```python
from build123d import *

# Parameters (mm, degrees)
SKETCH1_W           = 44
SKETCH1_H           = 29
BOSS_EXTRUDE1_DEPTH = 10.2
SKETCH2_W           = 8
SKETCH2_H           = 4
BOSS_EXTRUDE2_DEPTH = 4.3
FILLET1_R           = 3


with BuildPart() as part:
    # Sketch1 → Boss-Extrude1 (new body)
    with BuildSketch(Plane(origin=(0, 0, 0), x_dir=(1, 0, 0), z_dir=(0, 1, 0))):
        with Locations((22, 14.5)):
            Rectangle(SKETCH1_W, SKETCH1_H)
    extrude(amount=BOSS_EXTRUDE1_DEPTH)

    # Sketch2 → Boss-Extrude2 (add)
    with BuildSketch(Plane(origin=(0, 10.2, 0), x_dir=(1, 0, 0), z_dir=(0, 1, 0))):
        with Locations((28.5, 2)):
            Rectangle(SKETCH2_W, SKETCH2_H)
        with Locations((15.5, 2)):
            Rectangle(SKETCH2_W, SKETCH2_H)
    extrude(amount=BOSS_EXTRUDE2_DEPTH)

    # Fillet1
    fillet1_edges = [part.edges().sort_by_distance(p)[0] for p in [
        (0, 5.1, -29),
        (44, 5.1, -29),
        (44, 5.1, 0),
        (0, 5.1, 0),
    ]]
    fillet(fillet1_edges, radius=FILLET1_R)


solid = part.part
```
The model under review builds one solid part; all positions refer to its coordinate system, in mm. A direction names the side the tool comes from. Give positions to 0.01 mm unless a question says otherwise; leave off trailing zeros. Write each loop counter-clockwise with the first axis right and the second up, starting at its lowest first coordinate (ties: lowest second). Pieces come first, ordered by that corner, then holes. Notation, with made-up numbers: M 88.5,-9.75 L 118.5,-9.75 A17 cw 118.5,12.25 Z; hole C -36.5,-1.5 d7. An arc over 180 degrees is marked long. Answer in a Markdown table with one row per item.
Item 1: For P1, Ø1.2, axis at y = 12, z = -1.5, coming from the -X side; P2, Ø6, axis at x = 14.5, z = -7.5, coming from the +Y side; P3, Ø2, axis at x = 15.5, y = 12, coming from the -Z side, all flat-tipped, find the tip position at first contact; note any pin that passes through.
Check sheet entries:
| item | result |
|---|---|
| P1 | x = 11.5 |
| P2 | y = 10.2 |
| P3 | z = -4 |
Item 2: For line 1 along Y through (x, z) = (16, -14); line 2 along Z through (x, y) = (25, 11.75), list the stretches that pass through material, from the lowest coordinate up.
Check sheet entries:
| item | result |
|---|---|
| line 1 | 0 to 10.2 |
| line 2 | -4 to 0 |
Item 3: Add section B-B on x = 15.5. Give the boundary of the cut face in (y, z), plus the area to 3 significant figures.
Check sheet entries:
| item | result |
|---|---|
| outline | M 0,-29 L 10.2,-29 L 10.2,-4 L 14.5,-4 L 14.5,0 L 0,0 Z |
| area | 313 mm2 |
Item 4: Add section C-C on z = -11. Give the boundary of the cut face in (x, y).
Check sheet entries:
| item | result |
|---|---|
| outline | M 0,0 L 44,0 L 44,10.2 L 0,10.2 Z |
Item 5: Tool access review of faces 4 (the face through (43.1, 5.17, -28.14)), 5 (the face through (11.5, 12, -2)), 6 (the face through (32.5, 12, -2)), 7 (the face through (28, 12, -4)), 8 (the face through (24.5, 12, -2)): name each direction out of +Z, -Z, +X, -X, +Y, -Y from which nothing blocks a thin tool from reaching the whole face with its end or side.
Check sheet entries:
| item | result |
|---|---|
| face 4 | -Z, +X, +Y, -Y |
| face 5 | +Z, -Z, -X, +Y |
| face 6 | +Z, -Z, +X, +Y |
| face 7 | -Z, +X, -X, +Y |
| face 8 | +Z, -Z, +Y |
Item 6: Add section D-D on x = 40. Give the boundary of the cut face in (y, z).
Check sheet entries:
| item | result |
|---|---|
| outline | M 0,-29 L 10.2,-29 L 10.2,0 L 0,0 Z |
Item 7: Add section A-A on y = 12.25. Give the boundary of the cut face in (x, z).
Check sheet entries:
| item | result |
|---|---|
| outline | M 11.5,-4 L 19.5,-4 L 19.5,0 L 11.5,0 Z; M 24.5,-4 L 32.5,-4 L 32.5,0 L 24.5,0 Z |
Item 8: Draft analysis for pull direction X (two halves, no side actions). For faces 1 (the face through (0.86, 5.17, -28.1)), 2 (the face through (22, 0, -15)), 3 (the face through (19.5, 12, -2)), state which applies: +X half, -X half, draft (parallel to the pull), parting line (faces both ways), or undercut.
Check sheet entries:
| item | result |
|---|---|
| face 1 | -X half |
| face 2 | draft |
| face 3 | undercut |
